```python
from build123d import *

# Parameters (mm, degrees)
F0_W     = 150.715396
F0_H     = 70.35607
F1_DEPTH = 25
F2_R     = 5
F3_R     = 5
F5_D     = 20


with BuildPart() as f1:
    # F0 (on Top) → F1 (new body)
    with BuildSketch(Plane.XY):
        Rectangle(F0_W, F0_H)
    extrude(amount=F1_DEPTH)

    # F2
    f2_edges = [f1.edges().sort_by_distance(p)[0] for p in [
        (0, -35.178035, 25),
    ]]
    fillet(f2_edges, radius=F2_R)

    # F3
    f3_edges = [f1.edges().sort_by_distance(p)[0] for p in [
        (0, -35.178035, 0),
    ]]
    fillet(f3_edges, radius=F3_R)

    # F5 (through all)
    with Locations(Plane.XY.offset(25)):
        with Locations((0.679701, -3.219078)):
            Hole(F5_D / 2)


solid = f1.part
```
Build history of the part. All positions in model axes, mm. Give positions to 0.01 mm unless a question says otherwise; leave off trailing zeros. Loops run counter-clockwise (first coordinate to the right, second up) from the corner with the lowest first, then second, coordinate; pieces in that order, holes last. Notation, with made-up numbers: (30, 57.5) - (78, 57.5) arc R16 ccw to (78, 81.5) - close; hole circle Ø6 at (-6, -10.5). An arc over 180 degrees is marked (long way). Use a Markdown table: item, result.
(1) Band-saw the part on A-A (x = -3.5). Give the cut face in (y, z), and give its area (3 significant figures).
Taken from the geometry:
| item | result |
|---|---|
| outline | (-35.18, 5) arc R5 ccw to (-30.18, 0) - (-12.3, 0) - (-12.3, 25) - (-30.18, 25) arc R5 ccw to (-35.18, 20) - close; (5.87, 0) - (35.18, 0) - (35.18, 25) - (5.87, 25) - close |
| area | 1,290 mm2 |
(2) Band-saw the part on B-B (z = 10). Give the cut face in (x, y).
Taken from the geometry:
| item | result |
|---|---|
| outline | (-75.36, -35.18) - (75.36, -35.18) - (75.36, 35.18) - (-75.36, 35.18) - close; hole circle Ø20 at (0.68, -3.22) |
(3) Wall check: line 1 along X through (y, z) = (-2, 4.75); line 2 along X through (y, z) = (2, 19.5); line 3 along Y through (x, z) = (-7.5, 9.5). Give the ranges that are in metal, low to high.
Taken from the geometry:
| item | result |
|---|---|
| line 1 | -75.36 to -9.25, 10.61 to 75.36 |
| line 2 | -75.36 to -7.85, 9.21 to 75.36 |
| line 3 | -35.18 to -8.97, 2.53 to 35.18 |
(4) Band-saw the part on C-C (z = 3). Give the cut face in (x, y), and give its area (3 significant figures).
Taken from the geometry:
| item | result |
|---|---|
| outline | (-75.36, -34.76) - (75.36, -34.76) - (75.36, 35.18) - (-75.36, 35.18) - close; hole circle Ø20 at (0.68, -3.22) |
| area | 10,200 mm2 |
(5) Pull direction Y, two halves, no side cores. Call faces 1 (the face through (-8.86, -0.22, 12.32)), 2 (the face through (-1, -35.178, 12)), 3 (the face through (-1, 10, 25)): +Y half, -Y half, draft (parallel to the pull), parting line (faces both ways), or undercut.
Taken from the geometry:
| item | result |
|---|---|
| face 1 | undercut |
| face 2 | -Y half |
| face 3 | draft |
